from build123d import *

# Parameters (mm, degrees)
F2_R     = 0.7
F3_DEPTH = 4
F4_R     = 1


with BuildPart() as f1:
    # F0 (on Front) → F1 (revolve)
    with BuildSketch(Plane.XZ):
        Polygon((0, -1.1), (0, 0), (0, 20.9), (-1, 20.9), (-1, 13.4), (-3.25, 13.4), (-3.25, 12.4), (-12.15, 12.4), (-12.15, 0), (-1.966873, 0), (-1.966873, -1.1), align=None)
    revolve(axis=Axis((0, 0, 10.45), (0, 0, 1)))

    # F2 (on face) → F3 (cut)
    with BuildSketch(Plane.XY.offset(12.4)):
        with BuildLine():
            ThreePointArc((0, 7.55), (0.494975, 7.755025), (0.7, 8.25))
            ThreePointArc((0.7, 8.25), (-0.494975, 8.744975), (0, 7.55))
        make_face()
        with Locations((-7.14471, 4.125)):
            Circle(F2_R)
        with Locations((-7.14471, -4.125)):
            Circle(F2_R)
        with Locations((0, -8.25)):
            Circle(F2_R)
        with Locations((7.14471, -4.125)):
            Circle(F2_R)
        with Locations((7.14471, 4.125)):
            Circle(F2_R)
    extrude(amount=-F3_DEPTH, mode=Mode.SUBTRACT)

    # F4
    f4_edges = [f1.edges().sort_by_distance(p)[0] for p in [
        (12.15, 0, 12.4),
    ]]
    fillet(f4_edges, radius=F4_R)


solid = f1.part
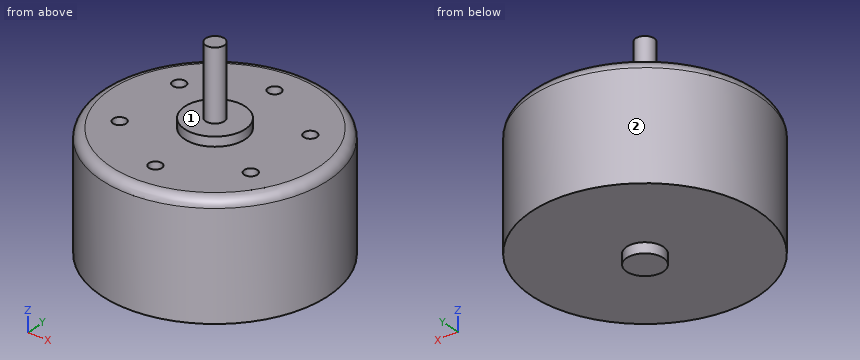
Design review of the part built by this model. Coordinates are the model's own, in mm. Face numbers are marked on the shaded views. A direction names the side the tool comes from. Round coordinates to 2 decimals unless told otherwise and drop trailing zeros. Write each loop counter-clockwise with the first axis right and the second up, starting at its lowest first coordinate (ties: lowest second). Pieces come first, ordered by that corner, then holes. Notation, with made-up numbers: (86, -5.75) - (113, -5.75) arc R23 ccw to (113, 21.25) - close; hole circle Ø10 at (38, 21). An arc over 180 degrees is marked (long way). Return JSON: item names as keys, results as strings. Group by question number.
Item 1: Machinability: for the marked faces 1 and 2, which of the approach directions +Z, -Z, +X, -X, +Y, -Y give a long, thin tool a straight path to every point of the face, cutting with its end or side? Answer none if there is none.
Item 2: We need section C-C on z = 2.5. Write out the cut boundary in (x, y).
Item 3: For probe 1 along Y at (x, z) = (0, 10.95); probe 2 along Z at (x, y) = (-6, 1.75); probe 3 along X at (y, z) = (3.5, 12.25), list the stretches that pass through material, from the lowest coordinate up. Write a range as [from, to].
Item 4: We need section A-A on z = 10. Write out the cut boundary in (x, y) (3 decimals), and give its area (3 significant figures).
Item 5: We need section B-B on y = 0. Write out the cut boundary in (x, z).
Item 6: Insertion check: P1, Ø0.7, axis at x = 0, y = -8, coming from the +Z side; P2, Ø2, axis at x = 1, y = -1, coming from the +Z side; P3, Ø6, axis at y = 8.5, z = 11, coming from the -X side; P4, Ø1.1, axis at x = -7.14, y = 4.12, coming from the -Z side. Each pin has a flat end and moves straight along its axis. Give the tip position at first contact, or say it passes through.
Item 7: We need section D-D on z = 16.5. Write out the cut boundary in (x, y), and give its area (3 significant figures).
Model answer:
{
 "1": {"face 1": "+Z", "face 2": "+Z, -Z"},
 "2": {"outline": "circle Ø24.3 at (0, 0)"},
 "3": {"probe 1": "y = [-12.15, -8.95], [-7.55, 7.55], [8.95, 12.15]", "probe 2": "z = [0, 12.4]", "probe 3": "x = [-11.14, -7.46], [-6.83, 6.83], [7.46, 11.14]"},
 "4": {"outline": "circle Ø24.3 at (0, 0); hole circle Ø1.4 at (-7.145, -4.125); hole circle Ø1.4 at (-7.145, 4.125); hole circle Ø1.4 at (0, -8.25); hole (0, 7.55) arc R0.7 ccw to (0.7, 8.25) arc R0.7 ccw (long way) to start; hole circle Ø1.4 at (7.145, -4.125); hole circle Ø1.4 at (7.145, 4.125)", "area": "455 mm²"},
 "5": {"outline": "(-12.15, 0) - (-1.97, 0) - (-1.97, -1.1) - (1.97, -1.1) - (1.97, 0) - (12.15, 0) - (12.15, 11.4) arc R1 ccw to (11.15, 12.4) - (3.25, 12.4) - (3.25, 13.4) - (1, 13.4) - (1, 20.9) - (-1, 20.9) - (-1, 13.4) - (-3.25, 13.4) - (-3.25, 12.4) - (-11.15, 12.4) arc R1 ccw to (-12.15, 11.4) - close"},
 "6": {"P1": "stops at z = 8.4", "P2": "stops at z = 20.9", "P3": "stops at x = -10.83", "P4": "stops at z = 0"},
 "7": {"outline": "circle Ø2 at (0, 0)", "area": "3.14 mm²"}
}
